Can you work these out from the model? Positions are in its coordinate system, mm. Give positions to 0.01 mm unless a question says otherwise; leave off trailing zeros. Order: outer loops, then holes, each group sorted by start corner. A loop starts at its lowest first (then second) coordinate and runs counter-clockwise, first axis right, second up. Notation, with made-up numbers: (86, 64.5) - (132, 64.5) arc R26 ccw to (132, 88.5) - close; hole circle Ø8 at (21.5, 9.25). An arc over 180 degrees is marked (long way). One line per question, with ' | ' between items.
Autodesk Inventor part; units mm, degrees
ref_plane "YZ Plane" through (0, 0, 0) normal (1, 0, 0) x (0, 1, 0)
ref_plane "XZ Plane" through (0, 0, 0) normal (0, 1, 0) x (-1, 0, 0)
ref_plane "XY Plane" through (0, 0, 0) normal (0, 0, 1) x (1, 0, 0)
sketch "Sketch1" plane through (0, 0, 0) normal (0, 1, 0) x (-1, 0, 0)
  point P0 (0, 0)
sketch "Sketch2" plane through (0, 0, 0) normal (0, 1, 0) x (-1, 0, 0)
  line L0 (0, 0) -> (-5, 0)
  line L1 (-5, 0) -> (-5, -4)
  line L2 (-5, -4) -> (0, -4)
  line L3 (0, -4) -> (0, 0)
  line L4 (0, 0) -> (-10, 0)
  line L5 (-10, 0) -> (-10, -15)
  line L6 (-10, -15) -> (0, -15)
  line L7 (0, -15) -> (0, 0)
  circle A0 centre (-2, -2) radius 2
  line L8 (-5, 0) -> (-2, 0)
  line L9 (-2, 0) -> (-2, -4)
  line L10 (-2, -4) -> (-5, -4)
  line L11 (-5, -4) -> (-5, 0)
  point P0 (0, -2)
  dimension "d0" = 5
  dimension "d1" = 4
  dimension "d2" = 10
  dimension "d3" = 15
sketch "Sketch3" plane through (0, 0, 0) normal (0, 1, 0) x (-1, 0, 0)
  line L0 (0, 0) -> (0, -4.0004)
  line L1 (0, -4.0004) -> (0, -2.0004)
  line L2 (0, -4.0004) -> (-2.5, -4.0004)
  dimension "d4" = 2
  dimension "d5" = 2.5
extrude "Extrusion1" add sketch "Sketch2" along normal blind 10 contours L3 A0 L0 | A0 L2 L1 L0 | L3 L2 A0 | L1 L2 L7 L6 L5 L4
sketch "Sketch4" plane through (2, 0, 0) normal (0, 0, 1) x (1, 0, 0)
  line L0 (8, 0) -> (8, 10)
  line L1 (8, 10) -> (-2, 10)
  line L2 (-2, 10) -> (-2, 0)
  line L3 (-2, 0) -> (8, 0)
  line L4 (8, 0) -> (8, 10)
extrude "Extrusion2" add sketch "Sketch4" along normal blind 3
sketch "Sketch5" plane through (0, 0, 0) normal (0, -1, 0) x (1, 0, 0)
  line L0 (0, -15) -> (0, -2)
  line L1 (0, -0.3956) -> (0, -3.6044)
  line L2 (0, -3.666) -> (0, -0.334)
  line L3 (0, -2) -> (0, 3)
  line L4 (0, -0.334) -> (0, -3.666)
  point P0 (0, 0)
sketch "Sketch6" plane through (0, 0, 0) normal (0, -1, 0) x (1, 0, 0)
  line L0 (0, -15) -> (0, -2)
  line L1 (0, -2) -> (0.9417, -2)
  line L2 (0.9417, -2) -> (0.9417, -0.5)
  line L3 (0.9417, -0.5) -> (0, -0.5)
  line L4 (0, -0.5) -> (0, -2)
  circle A0 centre (2, -2) radius 2
  line L5 (0, -2) -> (0.8653, -2)
  line L6 (0.8653, -2) -> (0.8653, -3.5)
  line L7 (0.8653, -3.5) -> (0, -3.5)
  line L8 (0, -3.5) -> (0, -2)
  point P0 (0, 0)
  dimension "d10" = 1.5
  dimension "d11" = 1.5
extrude "Extrusion3" cut sketch "Sketch6" against normal blind 20 contours L0 A0 L7 | L1 L6 L7 A0
sketch "Sketch7" plane through (0, 0, 0) normal (0, -1, 0) x (1, 0, 0)
  arc A0 (0.6771, -3.5) -> (0, -2) centre (2, -2) ccw
  line L0 (0, -2) -> (0.9289, -2)
  line L1 (0.9289, -2) -> (0.9289, -0.5)
  line L2 (0.9289, -0.5) -> (0, -0.5)
  line L3 (0, -0.5) -> (0, -2)
  point P0 (0, 0)
  point P1 (0.6771, -0.5)
  dimension "d14" = 1.5
extrude "Extrusion4" cut sketch "Sketch7" against normal blind 20 contours A0 L3 L2
sketch "Sketch8" plane through (0, 0, 0) normal (0, -1, 0) x (1, 0, 0)
  point P0 (0, 0)
(1) Imagine slicing it at A-A (x = 2). List the corners of the cut face in (y, z) for me.
Answer below:
outline: (0, -15) - (10, -15) - (10, -4) - (0, -4) - close; (0, 0) - (10, 0) - (10, 3) - (0, 3) - close
(2) Imagine slicing it at C-C (z = -2). List the corners of the cut face in (x, y) for me.
Answer below:
outline: (4, 0) - (10, 0) - (10, 10) - (4, 10) - close
(3) If I drill on line 1 (Z direction, x = 2, y = 4); line 2 (Z direction, x = 0.5, y = 4.5); line 3 (X direction, y = 4.25, z = -2), over which ranges is the centre line in solid material (lowest first)?
Answer below:
line 1: -15 to -4, 0 to 3 | line 2: -15 to -3.5, -0.5 to 3 | line 3: 4 to 10
(4) Imagine slicing it at B-B (y = 4.5). List the corners of the cut face in (x, z) for me, and give its area (3 significant figures).
Answer below:
outline: (0, -15) - (10, -15) - (10, 3) - (0, 3) - (0, -0.5) - (0.68, -0.5) arc R2 cw (long way) to (0.68, -3.5) - (0, -3.5) - close | area: 167 mm^2
(5) If we mould it in two halves opening along Z, with no side actions, what happens to faces 1 (the face through (4, 5, -2)), 2 (the face through (5, 5, -15)), 3 (the face through (5, 5, 3)), 4 (the face through (5, 10, -6))? For each: released by +Z, released by -Z, zero draft, split by the parting line, or undercut.
Answer below:
face 1: undercut | face 2: released by -Z | face 3: released by +Z | face 4: zero draft
(6) Will this pin go through, and if not, where does the flat tip stop? pin 1 (3 mm diameter, centred on x = 2, z = -2, fed in from -Y).
Answer below:
pin 1: through
